The model under review builds one solid part; all positions refer to its coordinate system, in mm. A direction names the side the tool comes from. Round coordinates to 2 decimals unless told otherwise and drop trailing zeros. Loops run counter-clockwise (first coordinate to the right, second up) from the corner with the lowest first, then second, coordinate; pieces in that order, holes last. Notation, with made-up numbers: M -16,77 L 37,77 A22 ccw 37,100 Z; hole C 74.5,-21.75 d5. An arc over 180 degrees is marked long. Return JSON: item names as keys, results as strings. Group by question number.
Q1. Clearance check with flat-ended pins moving along their axes: pin 1 Ø1.6 at (x, y) = (-3, 0.5) entering from -Z; pin 2 Ø1.6 at (x, z) = (-3.5, -140) entering from -Y. State where each tip first meets the part, or that it passes through.
Q2. Consider section A-A (z = 0). State the section outline as (x, y) points, and give its area (3 significant figures).
Q3. Consider section B-B (y = 37.5). State the section outline as (x, z) points.
Q4. To check wall thickness, follow line 1 along Z through (x, y) = (5.5, 51.5); line 2 along X through (y, z) = (1.15, 0); line 3 along Z through (x, y) = (-6.5, 23). State the ranges of each line that lie inside material, in increasing order.
Q5. For faces 4 (the face through (0, 46, -139.263)), 5 (the face through (0.41, 38.81, -140.28)), 6 (the face through (0, 2, 0)), 7 (the face through (0, 34, 5.737)), list the 3-axis set-ups (+Z, -Z, +X, -X, +Y, -Y) from which the entire face can be reached by the end or side of a thin tool; tool diameter is ignored.
Q6. Consider section D-D (y = 4.5). State the section outline as (x, z) points.
Q7. Consider section C-C (x = 0). State the section outline as (y, z) points, and give its area (3 significant figures).
Q8. Draft analysis for pull direction X (two halves, no side actions). For faces 1 (the face through (-4.396, 1.014, -1.593)), 2 (the face through (8.75, 66, -61)), 3 (the face through (0, 0, 0)), state which applies: pulls with the +X half, pulls with the -X half, needs draft (parallel to the pull), parting line crosses it, or undercut.
from build123d import *

# Parameters (mm, degrees)
SKETCH1_W                    = 17.5
SKETCH1_H                    = 10
BASE_FLANGE1_DEPTH           = 2
EDGE_FLANGE1_DEPTH           = 17.5
EDGE_FLANGE2_STRIP_W         = 9.4732
EDGE_FLANGE2_STRIP_H         = 2
EDGE_FLANGE2_STRIP_CUT_DEPTH = 17.5
EDGE_FLANGE2_DEPTH           = 17.5
EDGE_FLANGE3_STRIP_W         = 9.4732
EDGE_FLANGE3_STRIP_H         = 2
EDGE_FLANGE3_STRIP_CUT_DEPTH = 17.5
EDGE_FLANGE3_DEPTH           = 17.5
F_4_CLEARANCE_HOLE1_D        = 3.2639
F_4_CLEARANCE_HOLE1_DEPTH    = 2
F_4_CLEARANCE_HOLE1_TIP      = 0.980574487
CUT_EXTRUDE3_DEPTH           = 2
SKETCH25_R                   = 1.373100621
CUT_EXTRUDE4_DEPTH           = 2


# Sheet-metal steps are written as plain solids
with BuildPart() as part:
    # Sketch1 → Base-Flange1 (new body)
    with BuildSketch(Plane(origin=(0, 0, 0), x_dir=(1, 0, 0), z_dir=(0, 1, 0))):
        Rectangle(SKETCH1_W, SKETCH1_H)
    extrude(amount=BASE_FLANGE1_DEPTH)

    # Edge-Flange1 section (across the edge) → Edge-Flange1 (add)
    with BuildSketch(Plane(origin=(-8.75, 2, 5.7366), x_dir=(0, 0, -1), z_dir=(1, 0, 0))):
        with BuildLine():
            Line((-2, 0.7366), (-2, 65.5))
            Line((-2, 65.5), (0, 65.5))
            Line((0, 65.5), (0, 0.7366))
            ThreePointArc((0, 0.7366), (0.215745145, 0.215745145), (0.7366, 0))
            Line((0.7366, 0), (0.7366, -2))
            ThreePointArc((0.7366, -2), (-1.198468417, -1.198468417), (-2, 0.7366))
        make_face()
    extrude(amount=EDGE_FLANGE1_DEPTH)

    # Edge-Flange2 strip (across the edge) → Edge-Flange2 strip cut (cut)
    with BuildSketch(Plane(origin=(-8.75, 67.5, 5.7366), x_dir=(0, -1, 0), z_dir=(1, 0, 0))):
        with Locations((-2, -1)):
            Rectangle(EDGE_FLANGE2_STRIP_W, EDGE_FLANGE2_STRIP_H)
    extrude(amount=EDGE_FLANGE2_STRIP_CUT_DEPTH, mode=Mode.SUBTRACT)

    # Edge-Flange2 section (across the edge) → Edge-Flange2 (add)
    with BuildSketch(Plane(origin=(-8.75, 67.5, 5.7366), x_dir=(0, -1, 0), z_dir=(1, 0, 0))):
        with BuildLine():
            Line((0, 0.7366), (0, 147))
            Line((0, 147), (2, 147))
            Line((2, 147), (2, 0.7366))
            ThreePointArc((2, 0.7366), (2.215745145, 0.215745145), (2.7366, 0))
            Line((2.7366, 0), (2.7366, -2))
            ThreePointArc((2.7366, -2), (0.801531583, -1.198468417), (0, 0.7366))
        make_face()
    extrude(amount=EDGE_FLANGE2_DEPTH)

    # Edge-Flange3 strip (across the edge) → Edge-Flange3 strip cut (cut)
    with BuildSketch(Plane(origin=(-8.75, 65.5, -141.2634), x_dir=(0, 0, 1), z_dir=(1, 0, 0))):
        with Locations((-2, -1)):
            Rectangle(EDGE_FLANGE3_STRIP_W, EDGE_FLANGE3_STRIP_H)
    extrude(amount=EDGE_FLANGE3_STRIP_CUT_DEPTH, mode=Mode.SUBTRACT)

    # Edge-Flange3 section (across the edge) → Edge-Flange3 (add)
    with BuildSketch(Plane(origin=(-8.75, 65.5, -141.2634), x_dir=(0, 0, 1), z_dir=(1, 0, 0))):
        with BuildLine():
            Line((0, 0.7366), (0, 38))
            Line((0, 38), (2, 38))
            Line((2, 38), (2, 0.7366))
            ThreePointArc((2, 0.7366), (2.215745145, 0.215745145), (2.7366, 0))
            Line((2.7366, 0), (2.7366, -2))
            ThreePointArc((2.7366, -2), (0.801531583, -1.198468417), (0, 0.7366))
        make_face()
    extrude(amount=EDGE_FLANGE3_DEPTH)

    # #4 Clearance Hole1
    with Locations(Plane.XZ):
        with Locations((4.75, 0), (-4.75, 0)):
            Hole(F_4_CLEARANCE_HOLE1_D / 2, depth=F_4_CLEARANCE_HOLE1_DEPTH)
            with Locations((0, 0, -(F_4_CLEARANCE_HOLE1_DEPTH + F_4_CLEARANCE_HOLE1_TIP / 2))):  # 118° drill point
                Cone(0, F_4_CLEARANCE_HOLE1_D / 2, F_4_CLEARANCE_HOLE1_TIP, mode=Mode.SUBTRACT)

    # Sketch23 → Cut-Extrude3 (cut)
    with BuildSketch(Plane.XZ.offset(-65.5)):
        with BuildLine():
            Line((-1.65, -61.0268), (-1.65, -56.0268))
            ThreePointArc((-1.65, -56.0268), (0, -54.3768), (1.65, -56.0268))
            Line((1.65, -56.0268), (1.65, -61.0268))
            ThreePointArc((1.65, -61.0268), (0, -62.6768), (-1.65, -61.0268))
        make_face()
    extrude(amount=-CUT_EXTRUDE3_DEPTH, mode=Mode.SUBTRACT)

    # Sketch25 → Cut-Extrude4 (cut)
    with BuildSketch(Plane(origin=(0, 0, -141.2634), x_dir=(-1, 0, 0), z_dir=(0, 0, -1))):
        with Locations(Location((0, 37.5, 0), (0, 0, 90))):
            Circle(SKETCH25_R)
    extrude(amount=-CUT_EXTRUDE4_DEPTH, mode=Mode.SUBTRACT)


solid = part.part
Values:
{
 "1": {"pin 1": "stops at z = -5", "pin 2": "stops at y = 27.5"},
 "2": {"outline": "M -8.75,0 L -6.38,0 L -6.38,2 L -8.75,2 Z; M -8.75,65.5 L 8.75,65.5 L 8.75,67.5 L -8.75,67.5 Z; M -3.12,0 L 3.12,0 L 3.12,2 L -3.12,2 Z; M 6.38,0 L 8.75,0 L 8.75,2 L 6.38,2 Z", "area": "56.9 mm2"},
 "3": {"outline": "M -8.75,-141.26 L -1.37,-141.26 L -1.37,-139.26 L -8.75,-139.26 Z; M -8.75,5.74 L 8.75,5.74 L 8.75,7.74 L -8.75,7.74 Z; M 1.37,-141.26 L 8.75,-141.26 L 8.75,-139.26 L 1.37,-139.26 Z"},
 "4": {"line 1": "z = -141.26 to -139.26, 5.74 to 7.74", "line 2": "x = -8.75 to -6.38, -3.12 to 3.12, 6.38 to 8.75", "line 3": "z = 5.74 to 7.74"},
 "5": {"face 4": "+X, -X, -Y", "face 5": "-Z", "face 6": "-Z, +X, -X", "face 7": "+X, -X"},
 "6": {"outline": "M -8.75,5.74 L 8.75,5.74 L 8.75,7.74 L -8.75,7.74 Z"},
 "7": {"outline": "M 0,-5 L 2,-5 L 2,5 A0.74 cw 2.74,5.74 L 64.76,5.74 A0.74 cw 65.5,5 L 65.5,-54.38 L 67.5,-54.38 L 67.5,5 A2.74 ccw 64.76,7.74 L 2.74,7.74 A2.74 ccw 0,5 Z; M 27.5,-141.26 L 36.13,-141.26 L 36.13,-139.26 L 27.5,-139.26 Z; M 38.87,-141.26 L 64.76,-141.26 A2.74 ccw 67.5,-138.53 L 67.5,-62.68 L 65.5,-62.68 L 65.5,-138.53 A0.74 cw 64.76,-139.26 L 38.87,-139.26 Z", "area": "500 mm2"},
 "8": {"face 1": "undercut", "face 2": "pulls with the +X half", "face 3": "needs draft"}
}
